Part model, mm, in its own coordinate system. A direction names the side the tool comes from. Give positions to 0.01 mm unless a question says otherwise; leave off trailing zeros. Order: outer loops, then holes, each group sorted by start corner. A loop starts at its lowest first (then second) coordinate and runs counter-clockwise, first axis right, second up. Notation, with made-up numbers: (58.25, 15.25) - (87.25, 15.25) arc R21 ccw to (87.25, 19.25) - close; hole circle Ø8 at (73.25, -26.75). An arc over 180 degrees is marked (long way). Use a Markdown table: item, result. Add a question column.
from build123d import *
from OCP.BRepFilletAPI import BRepFilletAPI_MakeChamfer

# Parameters (mm, degrees)
SKETCH_1_W          = 9.8
SKETCH_1_H          = 11
SKETCH_1_W_2        = 8.6
SKETCH_1_H_2        = 6
SKETCH_1_R          = 1.25
SKETCH_1_H_3        = 10.75
EXTRUDE_1_DEPTH     = 10
SKETCH_3_R          = 2.25
CUT_EXTRUDE_2_DEPTH = 26.121218621
CUT_EXTRUDE_3_DEPTH = 4
FILLET_2_R          = 7.5
CHAMFER_1_SIZE      = 0.6
CHAMFER_1_SIZE2     = 0.346410162
FILLET_3_R          = 8
CHAMFER_3_SIZE      = 1
CHAMFER_3_SIZE2     = 1.732050808


with BuildPart() as part:
    # ｽｹｯﾁ1 → ﾎﾞｽ - 押し出し1 (new body)
    # profile 1 of 5: a face of its own
    with BuildSketch(Plane(origin=(0, 0, 0), x_dir=(1, 0, 0), z_dir=(0, 1, 0))):
        with Locations((0, 8.375)):
            Rectangle(SKETCH_1_W, SKETCH_1_H)
    # profile 2 of 5: a face of its own
    with BuildSketch(Plane(origin=(0, 0, 0), x_dir=(1, 0, 0), z_dir=(0, 1, 0))):
        with Locations((9.2, -0.125)):
            Rectangle(SKETCH_1_W_2, SKETCH_1_H_2)
        with Locations(Location((9.5, -0.125, 0), (0, 0, 270))):
            Circle(SKETCH_1_R, mode=Mode.SUBTRACT)
    # profile 3 of 5: a face of its own
    with BuildSketch(Plane(origin=(0, 0, 0), x_dir=(1, 0, 0), z_dir=(0, 1, 0))):
        with Locations((0, -0.125)):
            Rectangle(SKETCH_1_W, SKETCH_1_H_2)
    # profile 4 of 5: a face of its own
    with BuildSketch(Plane(origin=(0, 0, 0), x_dir=(1, 0, 0), z_dir=(0, 1, 0))):
        with Locations((-9.2, -0.125)):
            Rectangle(SKETCH_1_W_2, SKETCH_1_H_2)
        with Locations(Location((-9.5, -0.125, 0), (0, 0, 270))):
            Circle(SKETCH_1_R, mode=Mode.SUBTRACT)
    # profile 5 of 5: a face of its own
    with BuildSketch(Plane(origin=(0, 0, 0), x_dir=(1, 0, 0), z_dir=(0, 1, 0))):
        with Locations((0, -8.5)):
            Rectangle(SKETCH_1_W, SKETCH_1_H_3)
    extrude(amount=EXTRUDE_1_DEPTH)

    # ｽｹｯﾁ3 → ｶｯﾄ - 押し出し2 (cut, through all)
    with BuildSketch(Plane(origin=(4.9, 0, 0), x_dir=(0, 0, -1), z_dir=(1, 0, 0))):
        with Locations((-8.875, 5)):
            Circle(SKETCH_3_R)
    extrude(amount=-CUT_EXTRUDE_2_DEPTH, mode=Mode.SUBTRACT)

    # ｽｹｯﾁ5 → ｶｯﾄ - 押し出し3 (cut)
    with BuildSketch(Plane(origin=(0, 10, 0), x_dir=(1, 0, 0), z_dir=(0, 1, 0))):
        Polygon((4.9, 5), (2.508885395, 2.875), (-2.508885395, 2.875), (-4.9, 5), (-4.9, 2.875), (-7.025, 2.875), (-3.649308793, -0.125), (3.649308793, -0.125), (7.025, 2.875), (4.9, 2.875), align=None)
    extrude(amount=-CUT_EXTRUDE_3_DEPTH, mode=Mode.SUBTRACT)

    # ﾌｨﾚｯﾄ2
    fillet_2_edges = [part.edges().sort_by_distance(p)[0] for p in [
        (0, 0, 13.875),
    ]]
    fillet(fillet_2_edges, radius=FILLET_2_R)

    # 面取り1: one chamfer whose edges measure the first distance from different faces: ONE call of the kernel's chamfer builder (chamfer() names one face for all edges)
    chamfer_1_edges_1 = [part.edges().sort_by_distance(p)[0] for p in [
        (-10.2625, 10, -2.875),
        (-13.5, 10, 0.125),
        (-9.2, 10, 3.125),
        (-4.9, 10, 8.5),
        (0, 10, 13.875),
        (4.9, 10, 8.5),
        (9.2, 10, 3.125),
        (13.5, 10, 0.125),
        (10.2625, 10, -2.875),
        (-5.337154396, 10, -1.375),
        (0, 10, 0.125),
        (5.337154396, 10, -1.375),
        (9.5, 10, -1.125),
    ]]
    chamfer_1_side_1 = [part.faces().sort_by_distance(p)[0] for p in [
        (0, 10, 4.272957296),
    ]]
    chamfer_1_edges_2 = [part.edges().sort_by_distance(p)[0] for p in [
        (-4.9, 10, -9.4375),
        (4.9, 10, -9.4375),
        (0, 10, -13.875),
        (3.704442697, 10, -3.9375),
        (0, 10, -2.875),
        (-3.704442697, 10, -3.9375),
    ]]
    chamfer_1_side_2 = [part.faces().sort_by_distance(p)[0] for p in [
        (0, 10, -8.612025812),
    ]]
    chamfer_1_edges_3 = [part.edges().sort_by_distance(p)[0] for p in [
        (-9.5, 10, -1.125),
    ]]
    chamfer_1_side_3 = [part.faces().sort_by_distance(p)[0] for p in [
        (-9.5, 5, -1.125),
    ]]
    chamfer_1 = BRepFilletAPI_MakeChamfer(part.part.solid().wrapped)
    for e in chamfer_1_edges_1:
        chamfer_1.Add(CHAMFER_1_SIZE, CHAMFER_1_SIZE2, e.wrapped, chamfer_1_side_1[0].wrapped)  # the first distance lies on this face
    for e in chamfer_1_edges_2:
        chamfer_1.Add(CHAMFER_1_SIZE, CHAMFER_1_SIZE2, e.wrapped, chamfer_1_side_2[0].wrapped)  # the first distance lies on this face
    for e in chamfer_1_edges_3:
        chamfer_1.Add(CHAMFER_1_SIZE, CHAMFER_1_SIZE2, e.wrapped, chamfer_1_side_3[0].wrapped)  # the first distance lies on this face
    add(Compound.cast(chamfer_1.Shape()), mode=Mode.REPLACE)

    # ﾌｨﾚｯﾄ3
    # the kernel refuses this fillet: 8 mm, written as the material it adds along each edge
    with BuildSketch(Plane(origin=(-3.649308793, 17.256412491, 0.125), x_dir=(-0.7474768694815634, 0, -0.6642878364007891), z_dir=(0, -1, 0))) as fillet_3_piece_1_section:
        with BuildLine():
            CenterArc((FILLET_3_R * 0.380141132625, FILLET_3_R), FILLET_3_R, 228.372286683, 41.627713317)
            Line((-FILLET_3_R * 0.284146703776, FILLET_3_R * 0.252523130518), (0, 0))
            Line((0, 0), (FILLET_3_R * 0.380141132625, 0))
        make_face()
    fillet_3_piece_1 = extrude(amount=11.256412491, mode=Mode.PRIVATE)
    fillet_3_piece_1 = split(fillet_3_piece_1, bisect_by=Plane(origin=(-2.381035156, 9.533713371, -0.082632133), z_dir=(0, -0.8660254037844377, 0.5000000000000018)), keep=Keep.TOP, mode=Mode.PRIVATE)
    add(fillet_3_piece_1)
    with BuildSketch(Plane(origin=(-3.649308793, 17.256412491, 0.125), x_dir=(-0.7474768694815634, 0, -0.6642878364007891), z_dir=(0, -1, 0))) as fillet_3_piece_2_section:
        with BuildLine():
            CenterArc((FILLET_3_R * 0.380141132625, FILLET_3_R), FILLET_3_R, 228.372286683, 41.627713317)
            Line((-FILLET_3_R * 0.284146703776, FILLET_3_R * 0.252523130518), (0, 0))
            Line((0, 0), (FILLET_3_R * 0.380141132625, 0))
        make_face()
    fillet_3_piece_2 = extrude(amount=11.256412491, mode=Mode.PRIVATE)
    fillet_3_piece_2 = split(fillet_3_piece_2, bisect_by=Plane(origin=(-4.4593865, 9.533713371, -0.872698967), z_dir=(-0.3321439182003959, -0.8660254037844376, 0.37373843474078333)), keep=Keep.TOP, mode=Mode.PRIVATE)
    add(fillet_3_piece_2)
    with BuildSketch(Plane(origin=(3.649308793, 17.256412491, 0.125), x_dir=(0.7474768694815636, 0, -0.6642878364007891), z_dir=(0, -1, 0))) as fillet_3_piece_3_section:
        with BuildLine():
            CenterArc((FILLET_3_R * 0.380141132625, -FILLET_3_R), FILLET_3_R, 90, 41.627713317)
            Line((-FILLET_3_R * 0.284146703776, -FILLET_3_R * 0.252523130518), (0, 0))
            Line((0, 0), (FILLET_3_R * 0.380141132625, 0))
        make_face()
    fillet_3_piece_3 = extrude(amount=11.256412491, mode=Mode.PRIVATE)
    fillet_3_piece_3 = split(fillet_3_piece_3, bisect_by=Plane(origin=(2.381035156, 9.533713371, -0.082632133), z_dir=(0, -0.8660254037844377, 0.5000000000000018)), keep=Keep.TOP, mode=Mode.PRIVATE)
    add(fillet_3_piece_3)
    with BuildSketch(Plane(origin=(3.649308793, 17.256412491, 0.125), x_dir=(0.7474768694815636, 0, -0.6642878364007891), z_dir=(0, -1, 0))) as fillet_3_piece_4_section:
        with BuildLine():
            CenterArc((FILLET_3_R * 0.380141132625, -FILLET_3_R), FILLET_3_R, 90, 41.627713317)
            Line((-FILLET_3_R * 0.284146703776, -FILLET_3_R * 0.252523130518), (0, 0))
            Line((0, 0), (FILLET_3_R * 0.380141132625, 0))
        make_face()
    fillet_3_piece_4 = extrude(amount=11.256412491, mode=Mode.PRIVATE)
    fillet_3_piece_4 = split(fillet_3_piece_4, bisect_by=Plane(origin=(4.4593865, 9.533713371, -0.872698967), z_dir=(0.3321439182003956, -0.8660254037844377, 0.373738434740783)), keep=Keep.TOP, mode=Mode.PRIVATE)
    add(fillet_3_piece_4)
    # the kernel refuses this fillet: 8 mm, written as the material it takes off along each edge
    with BuildSketch(Plane(origin=(2.508885395, 17.256412491, -2.875), x_dir=(0.7474768694815637, 0, -0.664287836400789), z_dir=(0, -1, 0)), Plane(origin=(-2.508885395, 17.256412491, -2.875), x_dir=(1, 0, 0), z_dir=(0, -1, 0))) as fillet_3_2_piece_1:
        with BuildLine():
            CenterArc((FILLET_3_R * 0.380141132625, -FILLET_3_R), FILLET_3_R, 90, 41.627713317)
            Line((-FILLET_3_R * 0.284146703776, -FILLET_3_R * 0.252523130518), (0, 0))
            Line((0, 0), (FILLET_3_R * 0.380141132625, 0))
        make_face()
    extrude(amount=11.256412491, mode=Mode.SUBTRACT)

    # 面取り3
    chamfer_3_edges = [part.edges().sort_by_distance(p)[0] for p in [
        (9.2, 0, 3.125),
        (-9.2, 0, 3.125),
    ]]
    chamfer_3_side = [part.faces().sort_by_distance(p)[0] for p in [
        (0, 0, -2.510051578),
    ]]
    chamfer(chamfer_3_edges, length=CHAMFER_3_SIZE, length2=CHAMFER_3_SIZE2, reference=chamfer_3_side[0])


solid = part.part
1. Cut at C-C (z = 7.5). Write the cut outline in (x, y).
2. Pin check, flat tips, straight feed: P1, Ø5, axis at y = 7, z = -10, coming from the +X side; P2, Ø1, axis at x = -5.5, y = 3.5, coming from the +Z side (3 decimals); P3, Ø2.5, axis at x = -2.5, z = -2, coming from the +Y side; P4, Ø1.5, axis at x = -9.5, z = 0.125, coming from the +Y side. Stop position of each tip, or through.
3. Mould opens along Z. For faces 1 (the face through (0, 0, -4)), 2 (the face through (-9.26, 0.878, 2.632)), 3 (the face through (10.74, 4.76, -0.04)) say: released by +Z, released by -Z, zero draft, split by the parting line, or undercut.
4. Cut at B-B (y = 4.25). Write the cut outline in (x, z) (3 decimals).
5. Cut at D-D (z = -8.75). Write the cut outline in (x, y).
6. Drill centre lines: probe 1 along X at (y, z) = (9, 0.25); probe 2 along Z at (x, y) = (12, 4) (3 decimals); probe 3 along X at (y, z) = (7.25, 1). Where is each one in solid material? Low to high. Write a range as [from, to].
7. Cut at A-A (x = 9.5). Write the cut outline in (y, z) (3 decimals), plus the area to 3 significant figures.
8. Tool access for faces 4 (the face through (3.803, 9.863, -4.51)), 5 (the face through (9.14, 0.878, 2.632)), 6 (the face through (0, 6, -2)): list every direction of +Z, -Z, +X, -X, +Y, -Y with a clear straight run to the whole face (end or side of a thin tool).
Responses:
| question | item | result |
|---|---|---|
| 1 | outline | (-4.9, 0.08) - (4.9, 0.08) - (4.9, 3.22) - (-4.9, 3.22) - close; (-4.9, 6.78) - (4.9, 6.78) - (4.9, 9.65) - (4.3, 10) - (-4.3, 10) - (-4.9, 9.65) - close |
| 2 | P1 | stops at x = 4.9 |
| 2 | P2 | stops at z = 3.125 |
| 2 | P3 | stops at y = 6 |
| 2 | P4 | passes through |
| 3 | face 1 | zero draft |
| 3 | face 2 | released by +Z |
| 3 | face 3 | undercut |
| 4 | outline | (-13.5, -2.875) - (-4.9, -2.875) - (-4.9, -13.875) - (4.9, -13.875) - (4.9, -2.875) - (13.5, -2.875) - (13.5, 3.125) - (4.9, 3.125) - (4.9, 6.754) - (-4.9, 6.754) - (-4.9, 3.125) - (-13.5, 3.125) - close; (-4.9, 10.996) - (4.9, 10.996) - (4.9, 13.134) - (-4.9, 13.134) - close; hole circle Ø2.5 at (-9.5, 0.125); hole circle Ø2.5 at (9.5, 0.125) |
| 5 | outline | (-4.9, 0) - (4.9, 0) - (4.9, 9.65) - (4.3, 10) - (-4.3, 10) - (-4.9, 9.65) - close |
| 6 | probe 1 | x = [-13.5, -10.74], [-8.26, 8.26], [10.74, 13.5] |
| 6 | probe 2 | z = [-2.875, 3.125] |
| 6 | probe 3 | x = [-13.5, -10.39], [-8.61, 8.61], [10.39, 13.5] |
| 7 | outline | (0, -2.875) - (9.654, -2.875) - (10, -2.275) - (10, -1.725) - (9.654, -1.125) - (0, -1.125) - close; (0, 1.375) - (9.654, 1.375) - (10, 1.975) - (10, 2.525) - (9.654, 3.125) - (1.732, 3.125) - (0, 2.125) - close |
| 7 | area | 33.7 mm² |
| 8 | face 4 | +X, +Y |
| 8 | face 5 | +Z, +X, -Y |
| 8 | face 6 | +Y |
